Study the drawing (mm; zero at the part's minimum x, y, z) and answer. A direction names the side the tool comes from. Coordinates: 2 decimals unless noted, no trailing zeros. Loops run counter-clockwise (first coordinate to the right, second up) from the corner with the lowest first, then second, coordinate; pieces in that order, holes last.
Q1. Flat-ended cylindrical pins translate along their axes: P1, Ø3, axis at x = 18.5, z = 21.5, coming from the +Y side; P2, Ø5.5, axis at y = 2, z = 19, coming from the -X side; P3, Ø1.2, axis at x = 21.5, z = 29, coming from the +Y side. Find the tip coordinate at first contact, or state that the pin passes through.
Q2. Section D-D (x = 45) is taken. Give the vertices of the cut face in (y, z), then the cut area to 3 significant figures.
Q3. Section B-B (y = 6.25) is taken. Give the vertices of the cut face in (x, z), then the cut area to 3 significant figures.
Q4. Which of the six approach directions +Z, -Z, +X, -X, +Y, -Y give full straight-line access (tool end or side, diameter ignored) to the marked faces 5 and 6?
Q5. Straight lines are drawn through the part: line 1 (X direction, y = 3.9, z = 43); line 2 (Z direction, x = 82, y = 2); line 3 (Z direction, x = 64, y = 6). For each, find the intervals that lie inside material, in ascending order.
Q6. Section A-A (x = 6) is taken. Give the vertices of the cut face in (y, z).
Q7. The mould has two halves that part along Z. Classify the marked faces 1, 2, 3 and 4: pulls with the +Z half, pulls with the -Z half, needs draft (parallel to the pull), parting line crosses it, or undercut.
Q8. Section C-C (z = 24.5) is taken. Give the vertices of the cut face in (x, y).
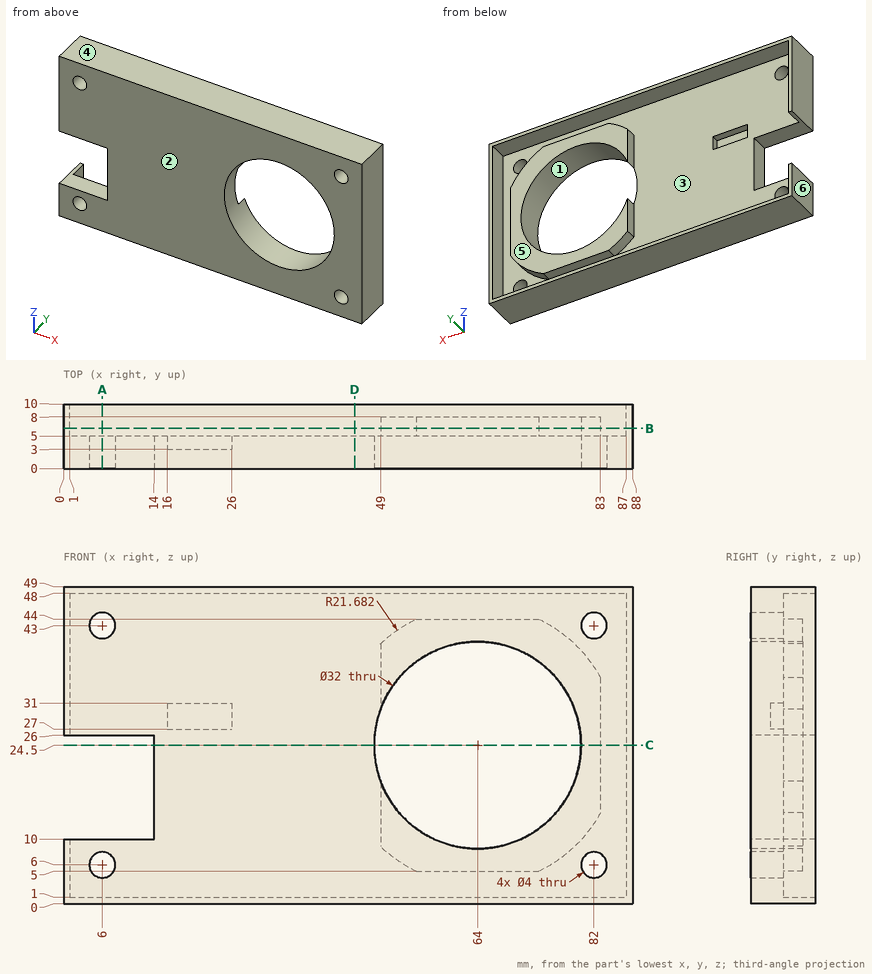
Numbers:
1. P1: stops at y = 5
1. P2: stops at x = 14
1. P3: stops at y = 3
2. outline: (0, 0) - (10, 0) - (10, 1) - (5, 1) - (5, 48) - (10, 48) - (10, 49) - (0, 49) - close
2. area: 255 mm2
3. outline: (0, 0) - (88, 0) - (88, 49) - (0, 49) - (0, 26) - (1, 26) - (1, 48) - (87, 48) - (87, 1) - (1, 1) - (1, 10) - (0, 10) - close; (49, 8.84) arc R21.68 ccw to (54.52, 5) - (73.48, 5) arc R21.68 ccw to (83, 14.05) - (83, 34.95) arc R21.68 ccw to (73.48, 44) - (54.52, 44) arc R21.68 ccw to (49, 40.16) - (49, 30.07) arc R16 cw (long way) to (49, 18.93) - close
3. area: 696 mm2
4. face 5: +Y
4. face 6: +Z, -Z, -X, +Y, -Y
5. line 1: x = 0 to 4, 8 to 80, 84 to 88
5. line 2: z = 0 to 4, 8 to 41, 45 to 49
5. line 3: z = 0 to 1, 5 to 8.5, 40.5 to 44, 48 to 49
6. outline: (0, 0) - (10, 0) - (10, 1) - (5, 1) - (5, 4) - (0, 4) - close; (0, 8) - (5, 8) - (5, 10) - (0, 10) - close; (0, 26) - (5, 26) - (5, 41) - (0, 41) - close; (0, 45) - (5, 45) - (5, 48) - (10, 48) - (10, 49) - (0, 49) - close
7. face 1: undercut
7. face 2: needs draft
7. face 3: undercut
7. face 4: pulls with the +Z half
8. outline: (14, 0) - (48, 0) - (48, 5) - (14, 5) - close; (80, 0) - (88, 0) - (88, 10) - (87, 10) - (87, 5) - (83, 5) - (83, 8) - (80, 8) - close
